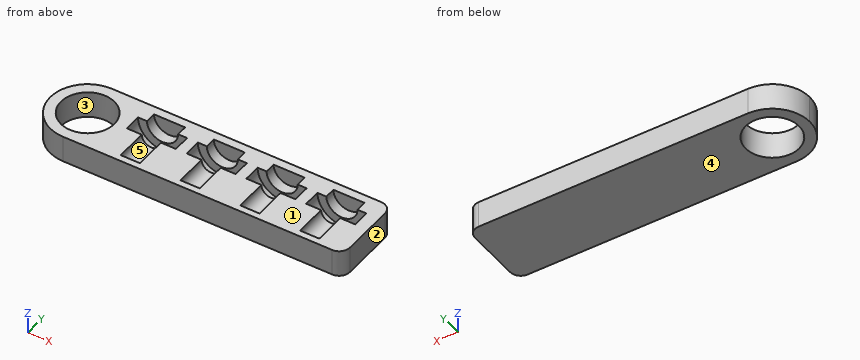
from build123d import *

# Parameters (mm, degrees)
F0_R     = 12.5
F1_DEPTH = 12.5


with BuildPart() as f1:
    # F0 (on Top) → F1 (new body)
    with BuildSketch(Plane.XY):
        with BuildLine():
            ThreePointArc((0, 17.5), (5.125631, 5.125631), (17.5, 0))
            Line((17.5, 0), (143.5, 0))
            ThreePointArc((143.5, 0), (147.035534, 1.464466), (148.5, 5))
            Line((148.5, 5), (148.5, 30))
            ThreePointArc((148.5, 30), (147.035534, 33.535534), (143.5, 35))
            Line((143.5, 35), (17.5, 35))
            ThreePointArc((17.5, 35), (5.125631, 29.874369), (0, 17.5))
        make_face()
        with Locations((17.5, 17.5)):
            Circle(F0_R, mode=Mode.SUBTRACT)
    extrude(amount=F1_DEPTH)

    # F2 (on face) → F3 (revolve, cut)
    with BuildSketch(Plane.XY.offset(12.5)):
        Polygon((47, 18), (47, 3), (51.5, 3), (51.5, 18), (58.5, 18), (58.5, 26), (54.3, 26), (54.3, 31), (47, 31), (47, 26), align=None)
    revolve(axis=Axis((47, 10.5, 12.5), (0, 1, 0)), mode=Mode.SUBTRACT)

    # F2 (on face) → F4 (revolve, cut)
    with BuildSketch(Plane.XY.offset(12.5)):
        Polygon((75, 18), (75, 3), (79.5, 3), (79.5, 18), (86.5, 18), (86.5, 26), (82.3, 26), (82.3, 31), (75, 31), (75, 26), align=None)
    revolve(axis=Axis((75, 22, 12.5), (0, 1, 0)), mode=Mode.SUBTRACT)

    # F2 (on face) → F5 (revolve, cut)
    with BuildSketch(Plane.XY.offset(12.5)):
        Polygon((103, 18), (103, 3), (107.5, 3), (107.5, 18), (114.5, 18), (114.5, 26), (110.3, 26), (110.3, 31), (103, 31), (103, 26), align=None)
    revolve(axis=Axis((103, 22, 12.5), (0, 1, 0)), mode=Mode.SUBTRACT)

    # F2 (on face) → F6 (revolve, cut)
    with BuildSketch(Plane.XY.offset(12.5)):
        Polygon((131, 18), (131, 3), (135.5, 3), (135.5, 18), (142.5, 18), (142.5, 26), (138.3, 26), (138.3, 31), (131, 31), (131, 26), align=None)
    revolve(axis=Axis((131, 22, 12.5), (0, 1, 0)), mode=Mode.SUBTRACT)


solid = f1.part
The listing builds one solid part. Answer for the finished solid, in the listing's coordinates (mm). Face numbers are marked on the shaded views. A direction names the side the tool comes from. Round coordinates to 2 decimals unless told otherwise and drop trailing zeros. Order: outer loops, then holes, each group sorted by start corner. A loop starts at its lowest first (then second) coordinate and runs counter-clockwise, first axis right, second up. Notation, with made-up numbers: (31, -11) -> (80, -11) arc R20 cw to (80, 7) -> close; hole circle Ø9 at (49.5, -28). An arc over 180 degrees is marked (long way). Put each result on its own line as item: value.
Q1. Section B-B, the plane x = 103 is taken. Write down the section's boundary in (y, z).
Results list:
outline: (0, 0) -> (35, 0) -> (35, 12.5) -> (31, 12.5) -> (31, 5.2) -> (26, 5.2) -> (26, 1) -> (18, 1) -> (18, 8) -> (3, 8) -> (3, 12.5) -> (0, 12.5) -> close
Q2. Consider line 1 along Y through (x, z) = (136.5, 2.5); line 2 along Y through (x, z) = (17.5, 6.75); line 3 along X through (y, z) = (25, 2.5). Determine where each line is inside the solid, lowest interval first.
Results list:
line 1: 0 to 18, 26 to 35
line 2: 0 to 5, 30 to 35
line 3: 1.69 to 7.5, 27.5 to 41.32, 52.68 to 69.32, 80.68 to 97.32, 108.68 to 125.32, 136.68 to 148.5
Q3. Section A-A, the plane z = 3.25 is taken. Write down the section's boundary in (x, y), and give its area (3 significant figures).
Results list:
outline: (0, 17.5) arc R17.5 ccw to (17.5, 0) -> (143.5, 0) arc R5 ccw to (148.5, 5) -> (148.5, 30) arc R5 ccw to (143.5, 35) -> (17.5, 35) arc R17.5 ccw to start; hole circle Ø25 at (17.5, 17.5); hole (40.17, 18) -> (53.83, 18) -> (53.83, 26) -> (40.17, 26) -> close; hole (68.17, 18) -> (81.83, 18) -> (81.83, 26) -> (68.17, 26) -> close; hole (96.17, 18) -> (109.83, 18) -> (109.83, 26) -> (96.17, 26) -> close; hole (124.17, 18) -> (137.83, 18) -> (137.83, 26) -> (124.17, 26) -> close
area: 4,130 mm^2
Q4. Section C-C, the plane x = 38 is taken. Write down the section's boundary in (y, z), and give its area (3 significant figures).
Results list:
outline: (0, 0) -> (35, 0) -> (35, 12.5) -> (26, 12.5) -> (26, 5.34) -> (18, 5.34) -> (18, 12.5) -> (0, 12.5) -> close
area: 380 mm^2
Q5. This flat-tipped pin is pushed along its axis until it touches: P1, Ø8, axis at x = 23.5, y = 13, coming from the -Z side. Where does it stop, or does it pass through?
Results list:
P1: through
Q6. Section D-D, the plane z = 11 is taken. Count the separate pieces of the cut face and the enclosed holes in it, and give its area (3 significant figures).
Results list:
separate pieces: 1
enclosed holes: 5
area: 3,040 mm^2
Q7. Which of the six approach directions +Z, -Z, +X, -X, +Y, -Y give full straight-line access (tool end or side, diameter ignored) to the marked faces 4 and 5?
Results list:
face 4: -Z, +X, -X, +Y, -Y
face 5: +Z
Q8. Determine the mould class of the marked faces 1, 2 and 3 for opening direction X: pulls with the +X half, pulls with the -X half, needs draft (parallel to the pull), parting line crosses it, or undercut.
Results list:
face 1: needs draft
face 2: pulls with the +X half
face 3: undercut
